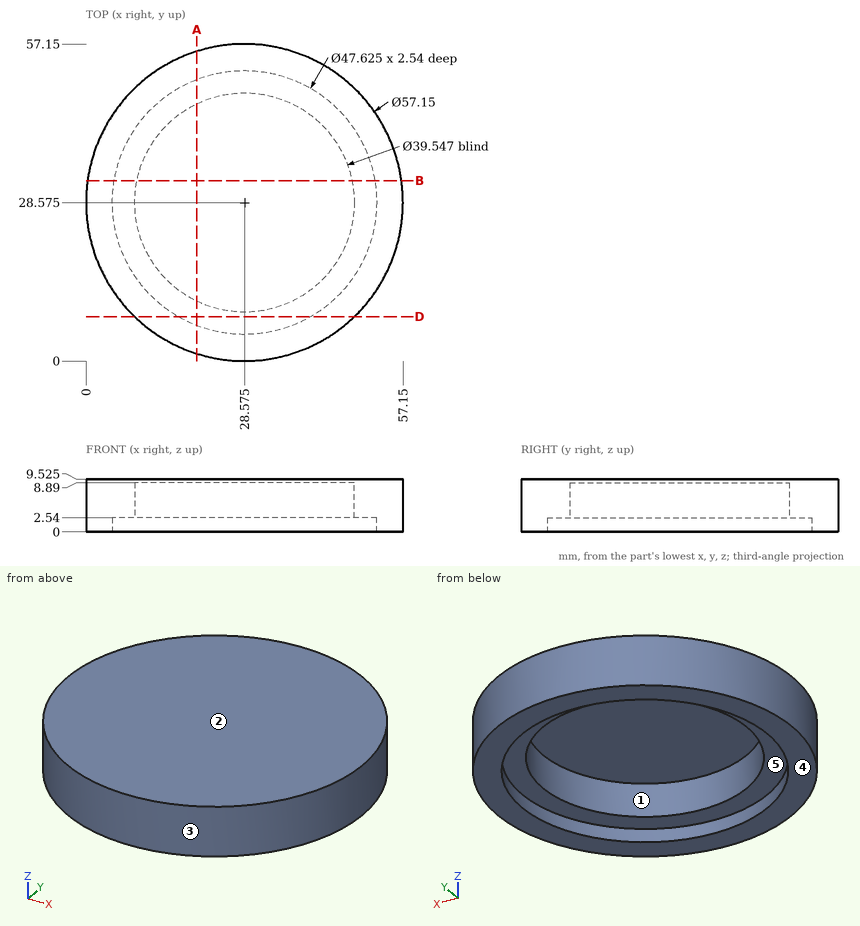
Check sheet for the drawn part. Datum: minimum x, y, z corner. Units: mm. A direction names the side the tool comes from. Round coordinates to 2 decimals unless told otherwise and drop trailing zeros. Loops run counter-clockwise (first coordinate to the right, second up) from the corner with the lowest first, then second, coordinate; pieces in that order, holes last.
Item 1: Thickness scan on line 1 (X direction, y = 39, z = 7.25); line 2 (X direction, y = 36, z = 8); line 3 (Y direction, x = 31.5, z = 0.75). Record the ranges inside material, lowest first.
Item 2: Gauge pin test, flat ends, axial feed: pin 1 (1.5 mm diameter, centred on y = 22.5, z = 2, fed in from -X); pin 2 (1 mm diameter, centred on x = 42.5, z = 1.5, fed in from -Y); pin 3 (3 mm diameter, centred on x = 20.5, y = 30.5, fed in from -Z). Record the tip position at first contact, or that the pin passes through.
Item 3: Cross-section at A-A on x = 20. Record the boundary of the cut face in (y, z) (1 decimal).
Item 4: Mould release check, pull along Y, two halves, no side actions. Record for the marked faces 1, 2 and 3: pulls with the +Y half, pulls with the -Y half, needs draft (parallel to the pull), parting line crosses it, or undercut.
Item 5: Access from +Z, -Z, +X, -X, +Y, -Y to the whole of each face (thin tool, end or side, straight path). Record for the marked faces 4 and 5.
Item 6: Cross-section at D-D on y = 8. Record the boundary of the cut face in (x, z) (1 decimal), then the cut area to 3 significant figures.
Item 7: Cross-section at B-B on y = 32.5. Record the boundary of the cut face in (x, z) (3 decimals).
Answer sheet:
1. line 1: x = 1.97 to 11.77, 45.38 to 55.18
1. line 2: x = 0.98 to 10.25, 46.9 to 56.17
1. line 3: y = 0.15 to 4.94, 52.21 to 57
2. pin 1: stops at x = 0.5
2. pin 2: stops at y = 3.35
2. pin 3: stops at z = 8.89
3. outline: (1.3, 0) - (6.4, 0) - (6.4, 2.5) - (10.8, 2.5) - (10.8, 8.9) - (46.4, 8.9) - (46.4, 2.5) - (50.8, 2.5) - (50.8, 0) - (55.8, 0) - (55.8, 9.5) - (1.3, 9.5) - close
4. face 1: undercut
4. face 2: needs draft
4. face 3: parting line crosses it
5. face 4: -Z, +X, -X, +Y, -Y
5. face 5: -Z
6. outline: (8.7, 0) - (16.6, 0) - (16.6, 2.5) - (40.6, 2.5) - (40.6, 0) - (48.4, 0) - (48.4, 9.5) - (8.7, 9.5) - close
6. area: 317 mm2
7. outline: (0.271, 0) - (5.088, 0) - (5.088, 2.54) - (9.195, 2.54) - (9.195, 8.89) - (47.955, 8.89) - (47.955, 2.54) - (52.062, 2.54) - (52.062, 0) - (56.879, 0) - (56.879, 9.525) - (0.271, 9.525) - close
